```python
from build123d import *

# Parameters (mm, degrees)
SKETCH1_R           = 1
BOSS_EXTRUDE1_DEPTH = 2
BOSS_EXTRUDE2_DEPTH = 1


with BuildPart() as part:
    # Sketch1 → Boss-Extrude1 (new body)
    with BuildSketch(Plane(origin=(0, 0, 0), x_dir=(1, 0, 0), z_dir=(0, 1, 0))):
        with BuildLine():
            Line((0, -2), (0, -3))
            Line((0, -3), (3, -3))
            Line((3, -3), (3, 3))
            Line((3, 3), (0, 3))
            ThreePointArc((0, 3), (-2.121320344, 2.121320344), (-3, 0))
            Line((-3, 0), (-2, 0))
            ThreePointArc((-2, 0), (-1.414213562, -1.414213562), (0, -2))
        make_face()
        Circle(SKETCH1_R, mode=Mode.SUBTRACT)
    extrude(amount=BOSS_EXTRUDE1_DEPTH)

    # Sketch3 → Boss-Extrude2 (add)
    with BuildSketch(Plane(origin=(3, 0, 0), x_dir=(0, 0, -1), z_dir=(1, 0, 0))):
        Polygon((0.996593321, 7), (2.996593321, 7), (2.996593321, 2), (-3, 2), (-3, 7), (-1.003406679, 7), (-1.003406679, 6), (0.996593321, 6), align=None)
    extrude(amount=-BOSS_EXTRUDE2_DEPTH)


solid = part.part
```
Verification items for the finished model (mm, model axes). A direction names the side the tool comes from. Coordinates: 2 decimals unless noted, no trailing zeros. Write each loop counter-clockwise with the first axis right and the second up, starting at its lowest first coordinate (ties: lowest second). Pieces come first, ordered by that corner, then holes. Notation, with made-up numbers: M 86,-25 L 118,-25 A22 ccw 118,-9 Z; hole C 84,48 d9. An arc over 180 degrees is marked long. Answer as a JSON object with one key per item and string values. Group by question number.
(1) Gauge pin test, flat ends, axial feed: pin 1 (0.8 mm diameter, centred on x = -2.5, y = 0.5, fed in from +Z); pin 2 (0.8 mm diameter, centred on x = 2.5, y = 4.5, fed in from -Z); pin 3 (0.8 mm diameter, centred on y = 1.5, z = 2.5, fed in from -X). Record the tip position at first contact, or that the pin passes through.
(2) Cross-section at B-B, the plane x = -0.4. Record the cut outline in (y, z).
(3) Release check for a two-part mould opening along X. For faces 5 (the face through (0, 1, 1)), 6 (the face through (0, 1, 2.5)), 7 (the face through (2.5, 4.5, -2.997)) record: +X half, -X half, draft (parallel to the pull), parting line (faces both ways), or undercut.
(4) Cross-section at A-A, the plane y = 1.25. Record the cut outline in (x, z).
(5) Material ranges on line 1 (X direction, y = 3.5, z = 0.15); line 2 (Y direction, x = 0.85, z = 2.65); line 3 (Z direction, x = 2.35, y = 6.5), recorded low to high.
(6) Tool access check on faces 1 (the face through (2.5, 6.5, 1.003)), 2 (the face through (2.5, 7, -2)), 3 (the face through (2, 5, 0)), 4 (the face through (-2.5, 1, 0)). Record the directions out of +Z, -Z, +X, -X, +Y, -Y that give a thin tool (end or side, any length) a straight path to the whole face; none if there is none.
(7) Cross-section at C-C, the plane z = -0.6. Record the cut outline in (x, y), and give its area (3 significant figures).
(8) Cross-section at D-D, the plane z = -1.65. Record the cut outline in (x, y), and give its area (3 significant figures).
Reply:
{
 "1": {"pin 1": "z = 0", "pin 2": "z = -3", "pin 3": "x = 0"},
 "2": {"outline": "M 0,-2.97 L 2,-2.97 L 2,-0.92 L 0,-0.92 Z; M 0,0.92 L 2,0.92 L 2,1.96 L 0,1.96 Z"},
 "3": {"face 5": "undercut", "face 6": "-X half", "face 7": "draft"},
 "4": {"outline": "M -3,0 A3 ccw 0,-3 L 3,-3 L 3,3 L 0,3 L 0,2 A2 ccw -2,0 Z; hole C 0,0 d2"},
 "5": {"line 1": "2 to 3", "line 2": "0 to 2", "line 3": "-3 to -1, 1 to 3"},
 "6": {"face 1": "+X, -X, +Y", "face 2": "+Z, -Z, +X, -X, +Y", "face 3": "+Z, -Z, -X, +Y", "face 4": "+Z, -X, +Y, -Y"},
 "7": {"outline": "M -2.94,0 L -0.8,0 L -0.8,2 L -2.94,2 Z; M 0.8,0 L 3,0 L 3,6 L 2,6 L 2,2 L 0.8,2 Z", "area": "12.7 mm²"},
 "8": {"outline": "M -2.51,0 L 3,0 L 3,7 L 2,7 L 2,2 L -2.51,2 Z", "area": "16.0 mm²"}
}
